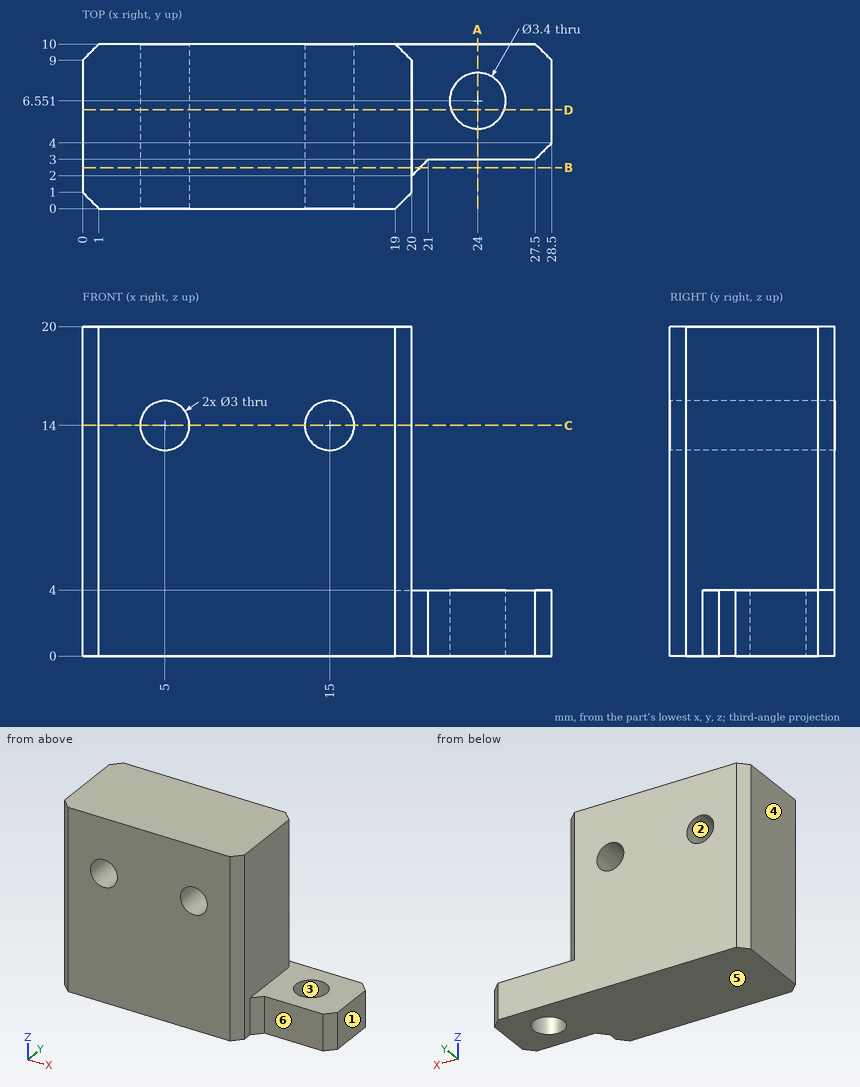
The figure shows three views and two pictorial views of one solid part (mm, origin at its lowest corner). Answer the questions. A direction names the side the tool comes from. Give positions to 0.01 mm unless a question says otherwise; leave off trailing zeros. Write each loop counter-clockwise with the first axis right and the second up, starting at its lowest first coordinate (ties: lowest second). Pieces come first, ordered by that corner, then holes. Notation, with made-up numbers: M 78.5,89.5 L 108.5,89.5 A14 cw 108.5,104.5 Z; hole C -36,49.5 d9. An arc over 180 degrees is marked long. One line per item, written item: value. Start each with the question number.
(1) Find section D-D (y = 6). Determine the outline of the cut face in (x, z).
(2) Find the intervals of material crossed by line 1 (Z direction, x = 15, y = 4.75); line 2 (X direction, y = 0.5, z = 15); line 3 (X direction, y = 3.25, z = 6.75), in increasing order.
(3) A tool of negligible diameter and unlimited length cuts with its end or side. For the marked faces 5 and 6, from which of +Z, -Z, +X, -X, +Y, -Y can it reach the whole face along a straight path? Write none if from no direction.
(4) Find section B-B (y = 2.5). Determine the outline of the cut face in (x, z), plus the area to 3 significant figures.
(5) Determine the mould class of the marked faces 1, 2, 3 and 4 for opening direction X: pulls with the +X half, pulls with the -X half, needs draft (parallel to the pull), parting line crosses it, or undercut.
(6) Flat-ended cylindrical pins translate along their axes: pin 1 Ø1 at (y, z) = (2.5, 17.5) entering from +X; pin 2 Ø1.5 at (x, z) = (22, 12.5) entering from +Y; pin 3 Ø3 at (x, z) = (24, 2.5) entering from -Y; pin 4 Ø4 at (x, y) = (24, 6.55) entering from +Z. Find the tip coordinate at first contact, or state that the pin passes through.
(7) Find section C-C (z = 14). Determine the outline of the cut face in (x, y).
(8) Find section A-A (x = 24). Determine the outline of the cut face in (y, z).
Results below:
1. outline: M 0,0 L 22.39,0 L 22.39,4 L 20,4 L 20,20 L 0,20 Z; M 25.61,0 L 28.5,0 L 28.5,4 L 25.61,4 Z; hole C 5,14 d3; hole C 15,14 d3
2. line 1: z = 0 to 12.5, 15.5 to 20
2. line 2: x = 0.5 to 3.88, 6.12 to 13.88, 16.12 to 19.5
2. line 3: x = 0 to 20
3. face 5: -Z, +X, -X, +Y, -Y
3. face 6: +Z, -Z, +X, -Y
4. outline: M 0,0 L 20.5,0 L 20.5,4 L 20,4 L 20,20 L 0,20 Z; hole C 5,14 d3; hole C 15,14 d3
4. area: 388 mm^2
5. face 1: pulls with the +X half
5. face 2: undercut
5. face 3: undercut
5. face 4: pulls with the -X half
6. pin 1: stops at x = 20
6. pin 2: passes through
6. pin 3: stops at y = 3
6. pin 4: stops at z = 4
7. outline: M 0,1 L 1,0 L 3.5,0 L 3.5,10 L 1,10 L 0,9 Z; M 6.5,0 L 13.5,0 L 13.5,10 L 6.5,10 Z; M 16.5,0 L 19,0 L 20,1 L 20,9 L 19,10 L 16.5,10 Z
8. outline: M 3,0 L 4.85,0 L 4.85,4 L 3,4 Z; M 8.25,0 L 10,0 L 10,4 L 8.25,4 Z
